Input: part model. Units: mm. Frame: model coordinates. Face numbers are marked on the shaded views. A direction names the side the tool comes from. Coordinates: 2 decimals unless noted, no trailing zeros. Order: outer loops, then holes, each group sorted by start corner. A loop starts at its lowest first (then second) coordinate and runs counter-clockwise, first axis right, second up. Notation, with made-up numbers: (48, -10.75) -> (62, -10.75) arc R36 cw to (62, 25.25) -> close; hole circle Ø9 at (32.5, 63). An arc over 180 degrees is marked (long way). Answer as CSV lines item,"result".
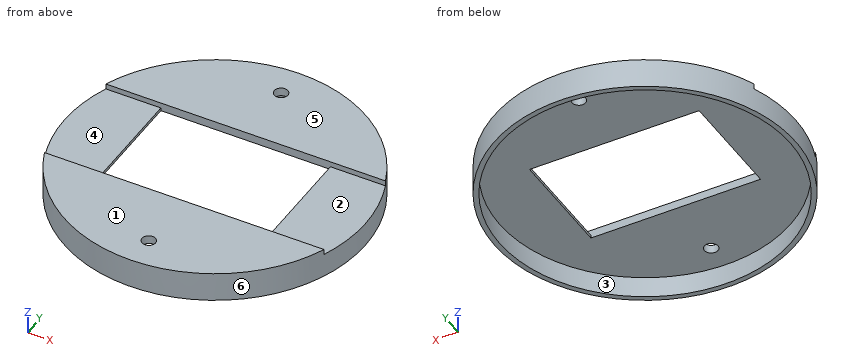
Autodesk Inventor part; units mm, degrees
ref_plane "YZ Plane" through (0, 0, 0) normal (1, 0, 0) x (0, 1, 0)
ref_plane "XZ Plane" through (0, 0, 0) normal (0, 1, 0) x (-1, 0, 0)
ref_plane "XY Plane" through (0, 0, 0) normal (0, 0, 1) x (1, 0, 0)
sketch "Sketch1" plane through (0, 0, 0) normal (0, 0, 1) x (1, 0, 0)
  circle A0 centre (0, 0) radius 34 construction
  circle A1 centre (0, 28) radius 1.6
  circle A2 centre (0, -28) radius 1.6
  circle A3 centre (0, 0) radius 34.25
  circle A4 centre (0, 0) radius 35.45
  dimension "d0" = 0.25
  dimension "d1" = 1.2
extrude "Extrusion1" add sketch "Sketch1" against normal blind 5 contours A4
sketch "Sketch4" plane through (0, 0, 0) normal (0, 0, 1) x (1, 0, 0)
  circle A0 centre (0, 0) radius 35.45
  circle A1 centre (0, 28) radius 1.6
  circle A2 centre (0, -28) radius 1.6
extrude "Extrusion2" add sketch "Sketch4" along normal blind 2
sketch "Sketch5" plane through (0, 0, 2) normal (0, 0, 1) x (1, 0, 0)
  circle A0 centre (0, 0) radius 35.45
  line L0 (-20, 13) -> (20, 13)
  line L1 (20, 13) -> (20, -13)
  line L2 (20, -13) -> (-20, -13)
  line L3 (-20, -13) -> (-20, 13)
  line L4 (-20, 13) -> (20, -13) construction
  line L5 (20, 13) -> (-20, -13) construction
  dimension "d6" = 40
  dimension "d7" = 26
extrude "Extrusion3" cut sketch "Sketch5" against normal through all contours L0 L1 L2 L3
sketch "Sketch6" plane through (0, 0, 2) normal (0, 0, 1) x (1, 0, 0)
  line L0 (32.2267, 13) -> (20, 13)
  line L1 (20, -13) -> (32.2267, -13)
  circle A0 centre (0, 0) radius 35.45
  circle A1 centre (0, 0) radius 35.45
  line L2 (32.9803, 13) -> (-32.9803, 13)
  line L3 (-20, 13) -> (20, 13)
  line L4 (32.9803, -13) -> (-32.9803, -13)
extrude "Extrusion4" cut sketch "Sketch6" against normal blind 1.3 contours L2 A0 L4 L1 L0
properties part number "LensMount_frame"
1. Contact query for flat-ended pins moving along their axis: pin 1 (3.5 mm diameter, centred on x = 0, y = 28, fed in from -Z); pin 2 (0.6 mm diameter, centred on x = 9.5, z = 1.5, fed in from -Y); pin 3 (12.5 mm diameter, centred on x = 26.5, y = 1, fed in from +Z). Output: stop coordinate, or through.
Findings:
pin 1,"stops at z = 0"
pin 2,"stops at y = -34.24"
pin 3,"stops at z = 0.7"
2. Cut plane C-C (x = -10.5). Return the cut outline in (y, z).
Findings:
outline,"(-33.86, -5) -> (-32.6, -5) -> (-32.6, 0) -> (-13, 0) -> (-13, 2) -> (-33.86, 2) -> close; (13, 0) -> (32.6, 0) -> (32.6, -5) -> (33.86, -5) -> (33.86, 2) -> (13, 2) -> close"
3. Reachability of the marked faces 1, 2 and 3 from +Z, -Z, +X, -X, +Y, -Y: full face, straight path, thin tool, end or side. Return the list, or none.
Findings:
face 1,"+Z, +X, -X, +Y, -Y"
face 2,"+Z, +X, -X"
face 3,"-Z"
4. Ray query, line 1 along Y through (x, z) = (0, 0.45); line 2 along Y through (x, z) = (0, -2.75); line 3 along Z through (x, y) = (-1.5, -18). Return the intervals inside material, ascending.
Findings:
line 1,"y = -35.45 to -29.6, -26.4 to -13, 13 to 26.4, 29.6 to 35.45"
line 2,"y = -35.45 to -34.25, 34.25 to 35.45"
line 3,"z = 0 to 2"
5. Cut plane B-B (x = 0). Return the cut outline in (y, z).
Findings:
outline,"(-35.45, -5) -> (-34.25, -5) -> (-34.25, 0) -> (-29.6, 0) -> (-29.6, 2) -> (-35.45, 2) -> close; (-26.4, 0) -> (-13, 0) -> (-13, 2) -> (-26.4, 2) -> close; (13, 0) -> (26.4, 0) -> (26.4, 2) -> (13, 2) -> close; (29.6, 0) -> (34.25, 0) -> (34.25, -5) -> (35.45, -5) -> (35.45, 2) -> (29.6, 2) -> close"
6. Cut plane D-D (y = 17.5). Return the cut outline in (x, z).
Findings:
outline,"(-30.83, -5) -> (-29.44, -5) -> (-29.44, 0) -> (29.44, 0) -> (29.44, -5) -> (30.83, -5) -> (30.83, 2) -> (-30.83, 2) -> close"
7. Cut plane A-A (y = 0). Return the cut outline in (x, z), plus the area to 3 significant figures.
Findings:
outline,"(-35.45, -5) -> (-34.25, -5) -> (-34.25, 0) -> (-20, 0) -> (-20, 0.7) -> (-35.45, 0.7) -> close; (20, 0) -> (34.25, 0) -> (34.25, -5) -> (35.45, -5) -> (35.45, 0.7) -> (20, 0.7) -> close"
area,"33.6 mm2"
8. Mould query, pull axis Y, two halves, no side actions, for the marked faces 4, 5 and 6. Classes: released by +Y, released by -Y, zero draft, split by the parting line, or undercut.
Findings:
face 4,"undercut"
face 5,"zero draft"
face 6,"split by the parting line"
